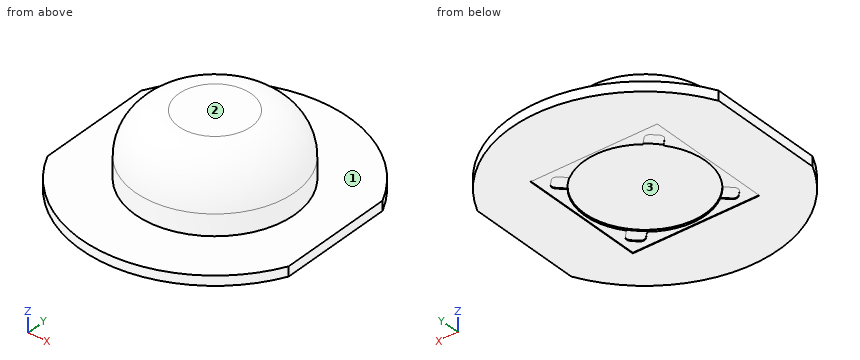
from build123d import *

# Parameters (mm, degrees)
BOSS_EXTRUDE1_DEPTH      = 4
SKETCH6_W                = 52.54
SKETCH6_H                = 52.54
CUT_EXTRUDE2_DEPTH       = 0.25
CUT_EXTRUDE3_DEPTH       = 0.3
CIRPATTERN1_COUNT        = 4
BOSS_EXTRUDE3_DEPTH      = 26.68
BOSS_EXTRUDE3_DEPTH_BACK = 3
SKETCH9_R                = 33.02
FILLET2_R                = 18


with BuildPart() as part:
    # Sketch1 → Boss-Extrude1 (new body)
    with BuildSketch(Plane.XY):
        with BuildLine():
            Line((50, 24.088378941), (50, -24.088378941))
            ThreePointArc((50, -24.088378941), (0, -55.5), (-50, -24.088378941))
            Line((-50, -24.088378941), (-50, 24.088378941))
            ThreePointArc((-50, 24.088378941), (0, 55.5), (50, 24.088378941))
        make_face()
    extrude(amount=BOSS_EXTRUDE1_DEPTH)

    # Sketch6 → Cut-Extrude2 (cut)
    with BuildSketch(Plane(origin=(0, 0, 0), x_dir=(-1, 0, 0), z_dir=(0, 0, -1))):
        Rectangle(SKETCH6_W, SKETCH6_H)
    extrude(amount=-CUT_EXTRUDE2_DEPTH, mode=Mode.SUBTRACT)

    # Sketch7 → Cut-Revolve1 (revolve, cut)
    with BuildSketch(Plane(origin=(0, 0, 0), x_dir=(1, 0, 0), z_dir=(0, 1, 0))):
        with BuildLine():
            Line((0, -0.25), (0, -25.25))
            ThreePointArc((0, -25.25), (17.67766953, -17.92766953), (25, -0.25))
            Line((25, -0.25), (0, -0.25))
        make_face()
    revolve(axis=Axis((0, 0, 0.25), (0, 0, 1)), mode=Mode.SUBTRACT)

    # Sketch8 → Cut-Extrude3 (cut)
    with BuildSketch(Plane(origin=(0, 0, 0.25), x_dir=(-1, 0, 0), z_dir=(0, 0, -1))):
        with BuildLine():
            Line((-19.887048211, -15.149432777), (-15.149432777, -19.887048211))
            Line((-15.149432777, -19.887048211), (-17.801083206, -22.53869864))
            ThreePointArc((-17.801083206, -22.53869864), (-19.215296769, -23.124485078), (-20.629510331, -22.53869864))
            Line((-20.629510331, -22.53869864), (-22.53869864, -20.629510331))
            ThreePointArc((-22.53869864, -20.629510331), (-23.124485078, -19.215296769), (-22.53869864, -17.801083206))
            Line((-22.53869864, -17.801083206), (-19.887048211, -15.149432777))
        make_face()
    cut_extrude3 = extrude(amount=-CUT_EXTRUDE3_DEPTH, mode=Mode.SUBTRACT)

    # CirPattern1: Cut-Extrude3 ×4 about axis
    cirpattern1_axis = Axis((0, 0, 0), (0, 0, 1))
    for i in range(1, CIRPATTERN1_COUNT):
        add(cut_extrude3.rotate(cirpattern1_axis, i * 360 / CIRPATTERN1_COUNT), mode=Mode.SUBTRACT)

    # Sketch9 → Boss-Extrude3 (add, two sides: drawn at the far end of the back side and taken through both)
    with BuildSketch(Plane.XY.offset(4).offset(-BOSS_EXTRUDE3_DEPTH_BACK)):
        Circle(SKETCH9_R)
    extrude(amount=BOSS_EXTRUDE3_DEPTH + BOSS_EXTRUDE3_DEPTH_BACK)

    # Fillet2
    fillet2_edges = [part.edges().sort_by_distance(p)[0] for p in [
        (-33.02, 0, 30.68),
    ]]
    fillet(fillet2_edges, radius=FILLET2_R)


solid = part.part
The listing builds one solid part. Answer for the finished solid, in the listing's coordinates (mm). Face numbers are marked on the shaded views. A direction names the side the tool comes from. Give positions to 0.01 mm unless a question says otherwise; leave off trailing zeros. Write each loop counter-clockwise with the first axis right and the second up, starting at its lowest first coordinate (ties: lowest second). Pieces come first, ordered by that corner, then holes. Notation, with made-up numbers: (53, 32.25) - (62, 32.25) arc R17 ccw to (62, 59.25) - close; hole circle Ø7 at (-8, 47.5). An arc over 180 degrees is marked (long way). Use a Markdown table: item, result.
1. A tool of negligible diameter and unlimited length cuts with its end or side. For the marked faces 1, 2 and 3, from which of +Z, -Z, +X, -X, +Y, -Y can it reach the whole face along a straight path? Write none if from no direction.
Values follow:
| item | result |
|---|---|
| face 1 | +Z |
| face 2 | +Z, +X, -X, +Y, -Y |
| face 3 | -Z |
2. Find the intervals of material crossed by probe 1 along Z at (x, y) = (-11, -46); probe 2 along X at (y, z) = (-20, 10.5); probe 3 along Z at (x, y) = (25, -25), in increasing order. Write a range as from..to.
Values follow:
| item | result |
|---|---|
| probe 1 | z = 0..4 |
| probe 2 | x = -26.27..26.27 |
| probe 3 | z = 0.25..4 |
3. Section C-C on y = -43 is taken. Write down the section's boundary in (x, z), plus the area to 3 significant figures.
Values follow:
| item | result |
|---|---|
| outline | (-35.09, 0) - (35.09, 0) - (35.09, 4) - (-35.09, 4) - close |
| area | 281 mm² |
4. Each of these flat-tipped pins is pushed along its axis until it touches: P1, Ø12, axis at x = -7.5, y = 5.5, coming from the -Z side; P2, Ø2.5, axis at x = -17.5, y = -19.5, coming from the -Z side; P3, Ø8, axis at y = 19.5, z = 23.5, coming from the +X side. Where does it stop, or does it pass through?
Values follow:
| item | result |
|---|---|
| P1 | stops at z = 1 |
| P2 | stops at z = 0.55 |
| P3 | stops at x = 26.31 |
5. Section A-A on z = 6 is taken. Write down the section's boundary in (x, y), plus the area to 3 significant figures.
Values follow:
| item | result |
|---|---|
| outline | circle Ø66.04 at (0, 0) |
| area | 3,430 mm² |
6. Section B-B on x = 43.5 is taken. Write down the section's boundary in (y, z).
Values follow:
| item | result |
|---|---|
| outline | (-34.47, 0) - (34.47, 0) - (34.47, 4) - (-34.47, 4) - close |
